```python
from build123d import *

# Parameters (mm, degrees)
SKETCH1_R                = 14
BOSS_EXTRUDE1_DEPTH      = 10
SKETCH2_R                = 2.25
CUT_EXTRUDE1_DEPTH       = 5
SKETCH3_R                = 5
CUT_EXTRUDE2_DEPTH       = 1.8
SKETCH11_R               = 4
BOSS_EXTRUDE2_DEPTH      = 45.5
ESBO_O2_R                = 5
RESSALTO_EXTRUS_O1_DEPTH = 1.8


with BuildPart() as part:
    # Sketch1 → Boss-Extrude1 (new body)
    with BuildSketch(Plane.XY):
        Circle(SKETCH1_R)
    extrude(amount=BOSS_EXTRUDE1_DEPTH)

    # Sketch2 → Cut-Extrude1 (cut)
    with BuildSketch(Plane(origin=(0, 0, 0), x_dir=(-1, 0, 0), z_dir=(0, 0, -1))):
        Circle(SKETCH2_R)
    extrude(amount=-CUT_EXTRUDE1_DEPTH, mode=Mode.SUBTRACT)

    # Sketch3 → Cut-Extrude2 (cut)
    with BuildSketch(Plane(origin=(0, 0, 0), x_dir=(-1, 0, 0), z_dir=(0, 0, -1))):
        Circle(SKETCH3_R)
    extrude(amount=-CUT_EXTRUDE2_DEPTH, mode=Mode.SUBTRACT)

    # Sketch11 → Boss-Extrude2 (add)
    with BuildSketch(Plane.XY.offset(10)):
        Circle(SKETCH11_R)
    extrude(amount=BOSS_EXTRUDE2_DEPTH)

    # Esboço2 → Ressalto-extrusão1 (add)
    with BuildSketch(Plane.XY.offset(55.5)):
        with Locations(Location((0, 0, 0), (0, 0, 180))):
            Circle(ESBO_O2_R)
    extrude(amount=RESSALTO_EXTRUS_O1_DEPTH)


solid = part.part
```
The listing builds one solid part. Answer for the finished solid, in the listing's coordinates (mm). A direction names the side the tool comes from. Coordinates: 2 decimals unless noted, no trailing zeros. Write each loop counter-clockwise with the first axis right and the second up, starting at its lowest first coordinate (ties: lowest second). Pieces come first, ordered by that corner, then holes. Notation, with made-up numbers: (32, 8) -> (49, 8) arc R30 cw to (49, 32) -> close; hole circle Ø10 at (2, 71.25). An arc over 180 degrees is marked (long way). Write each question's results on one line, items separated by ' | '. Start each with the question number.
1) A cutting plane is placed at A-A (y = 0). Determine the outline of the cut face in (x, z), then the cut area to 3 significant figures.
2) Straight lines are drawn through the part: probe 1 along Y at (x, z) = (0, 0.45); probe 2 along Y at (x, z) = (0, 4.3); probe 3 along Z at (x, y) = (7, 11). For each, find the intervals that lie inside material, in ascending order.
3) A tool of negligible diameter and unlimited length cuts with its end or side. For faces 4 (the cylindrical face through (0.29, 2.23, 3.38)), 5 (the cylindrical face through (5, 0, 56)), 6 (the cylindrical face through (12.932, -5.362, 4.93)), from which of +Z, -Z, +X, -X, +Y, -Y can it reach the whole face along a straight path? Write none if from no direction.
4) A cutting plane is placed at D-D (y = -6). Determine the outline of the cut face in (x, z), then the cut area to 3 significant figures.
5) Flat-ended cylindrical pins translate along their axes: pin 1 Ø2 at (y, z) = (-1.5, 31) entering from -X; pin 2 Ø5 at (x, y) = (-9, -10) entering from +Z; pin 3 Ø1.3 at (x, y) = (-0.5, -0.5) entering from -Z; pin 4 Ø6 at (x, z) = (-8, 18.5) entering from +Y. Find the tip coordinate at first contact, or state that the pin passes through.
6) A cutting plane is placed at C-C (z = 38). Determine the outline of the cut face in (x, y), then the cut area to 3 significant figures.
7) For a pull along Y with two mould halves and no side action, classify faces 1 (the flat face through (-2.2, -1, 1.8)), 2 (the cylindrical face through (-0.867, -3.905, 32.432)), 3 (the flat face through (0, 0, 57.3)) as +Y half, -Y half, draft (parallel to the pull), parting line (faces both ways), or undercut.
Values follow:
1) outline: (-14, 0) -> (-5, 0) -> (-5, 1.8) -> (-2.25, 1.8) -> (-2.25, 5) -> (2.25, 5) -> (2.25, 1.8) -> (5, 1.8) -> (5, 0) -> (14, 0) -> (14, 10) -> (4, 10) -> (4, 55.5) -> (5, 55.5) -> (5, 57.3) -> (-5, 57.3) -> (-5, 55.5) -> (-4, 55.5) -> (-4, 10) -> (-14, 10) -> close | area: 630 mm²
2) probe 1: -14 to -5, 5 to 14 | probe 2: -14 to -2.25, 2.25 to 14 | probe 3: 0 to 10
3) face 4: -Z | face 5: +Z | face 6: +Z, -Z
4) outline: (-12.65, 0) -> (12.65, 0) -> (12.65, 10) -> (-12.65, 10) -> close | area: 253 mm²
5) pin 1: x = -3.97 | pin 2: z = 10 | pin 3: z = 5 | pin 4: through
6) outline: circle Ø8 at (0, 0) | area: 50.3 mm²
7) face 1: undercut | face 2: parting line | face 3: draft
